The model under review builds one solid part; all positions refer to its coordinate system, in mm. A direction names the side the tool comes from. Coordinates: 2 decimals unless noted, no trailing zeros. Write each loop counter-clockwise with the first axis right and the second up, starting at its lowest first coordinate (ties: lowest second). Pieces come first, ordered by that corner, then holes.
1) Machinability: for faces 4 (the flat face through (70, 25, 8)), 5 (the flat face through (-8, 25, 70)), 6 (the flat face through (8, 25, -70)), 7 (the cylindrical face through (-57, 32, 0)), which of the approach directions +Z, -Z, +X, -X, +Y, -Y give a long, thin tool a straight path to every point of the face, cutting with its end or side? Answer none if there is none.
2) For P1, Ø10, axis at x = -51.5, y = 37.5, coming from the +Z side; P2, Ø3, axis at x = -57.5, y = 36.5, coming from the +Z side; P3, Ø4, axis at x = 14.5, y = 31, coming from the -Z side, all flat-tipped, find the tip position at first contact; note any pin that passes through.
3) Mouldability with a two-part tool opening along X and no side actions: class faces 1 (the cylindrical face through (79.845, 22.185, -41.53)), 2 (the flat face through (62, 42, -18.75)), 3 (the cylindrical face through (-19.524, 18.759, -4.336)) as released by +X, released by -X, zero draft, split by the parting line, or undercut.
4) Add section C-C, the plane z = 1. State the section outline as (x, y) points, then the cut area to 3 significant figures.
5) Add section A-A, the plane x = 0. State the section outline as (y, z) points, then the cut area to 3 significant figures.
6) Add section B-B, the plane y = 12. State the section outline as (x, z) points, then the cut area to 3 significant figures.
7) For line 1 (X direction, y = 9, z = 0); line 2 (X direction, y = 28, z = 0); line 3 (Z direction, x = 0, y = 40), list the stretches that pass through material, from the lowest coordinate up.
8) Add section D-D, the plane y = 32. State the section outline as (x, z) points, then the cut area to 3 significant figures.
from build123d import *

# Parameters (mm, degrees)
ESQUISSE1_R                  = 90
BOSS_EXTRU_1_DEPTH           = 45
ESQUISSE2_R                  = 9
ENL_V_MAT_EXTRU_1_DEPTH      = 45
ESQUISSE2_3_R                = 9
ENL_V_MAT_EXTRU_2_DEPTH      = 20
ENL_V_MAT_EXTRU_3_DEPTH      = 18.75
R_P_TITION_CIRCULAIRE2_COUNT = 4
ESQUISSE4_R                  = 30
ENL_V_MAT_EXTRU_4_DEPTH      = 8
ESQUISSE4_3_R                = 20
ENL_V_MAT_EXTRU_5_DEPTH      = 136


with BuildPart() as part:
    # Esquisse1 → Boss.-Extru.1 (new body)
    with BuildSketch(Plane(origin=(0, 0, 0), x_dir=(1, 0, 0), z_dir=(0, 1, 0))):
        with Locations(Location((0, 0, 0), (0, 0, 90))):
            Circle(ESQUISSE1_R)
    extrude(amount=BOSS_EXTRU_1_DEPTH)

    # Esquisse2 → Enl_v. mat.-Extru.1 (cut)
    with BuildSketch(Plane(origin=(0, 45, 0), x_dir=(1, 0, 0), z_dir=(0, 1, 0))):
        with Locations(Location((75, 0, 0), (0, 0, 270))):
            Circle(ESQUISSE2_R)
    enl_v_mat_extru_1 = extrude(amount=-ENL_V_MAT_EXTRU_1_DEPTH, mode=Mode.SUBTRACT)

    # Esquisse2_3 → Enl_v. mat.-Extru.2 (cut)
    with BuildSketch(Plane(origin=(0, 45, 0), x_dir=(1, 0, 0), z_dir=(0, 1, 0))):
        with BuildLine():
            Line((75, 18), (115, 18))
            ThreePointArc((115, 18), (133, 0), (115, -18))
            Line((115, -18), (75, -18))
            ThreePointArc((75, -18), (57, 0), (75, 18))
        make_face()
        with Locations(Location((75, 0, 0), (0, 0, 270))):
            Circle(ESQUISSE2_3_R, mode=Mode.SUBTRACT)
    enl_v_mat_extru_2 = extrude(amount=-ENL_V_MAT_EXTRU_2_DEPTH, mode=Mode.SUBTRACT)

    # Esquisse3 → Enl_v. mat.-Extru.3 (cut, symmetric)
    with BuildSketch(Plane.XY):
        Polygon((-0.90918463, 45), (101.87081537, 35.103411626), (101.87081537, 45), align=None)
    enl_v_mat_extru_3 = extrude(amount=ENL_V_MAT_EXTRU_3_DEPTH, both=True, mode=Mode.SUBTRACT)

    # Sym_trie1: Enl_v. mat.-Extru.3 across plane
    add(enl_v_mat_extru_3.mirror(Plane(origin=(0, 0, 0), x_dir=(0, 0, 1), z_dir=(1, 0, 0))), mode=Mode.SUBTRACT)

    # R_p_tition circulaire2: Enl_v. mat.-Extru.1, Enl_v. mat.-Extru.2 ×4 about axis
    r_p_tition_circulaire2_axis = Axis((0, 0, 0), (0, 1, 0))
    add([enl_v_mat_extru_1.rotate(r_p_tition_circulaire2_axis, i * 360 / R_P_TITION_CIRCULAIRE2_COUNT) for i in range(1, R_P_TITION_CIRCULAIRE2_COUNT)], mode=Mode.SUBTRACT)
    add([enl_v_mat_extru_2.rotate(r_p_tition_circulaire2_axis, i * 360 / R_P_TITION_CIRCULAIRE2_COUNT) for i in range(1, R_P_TITION_CIRCULAIRE2_COUNT)], mode=Mode.SUBTRACT)

    # Esquisse4 → Enl_v. mat.-Extru.4 (cut, symmetric)
    with BuildSketch(Plane(origin=(0, 45, 0), x_dir=(1, 0, 0), z_dir=(0, 1, 0))):
        with Locations(Location((0, 0, 0), (0, 0, 270))):
            Circle(ESQUISSE4_R)
    extrude(amount=ENL_V_MAT_EXTRU_4_DEPTH, both=True, mode=Mode.SUBTRACT)

    # Esquisse4_3 → Enl_v. mat.-Extru.5 (cut, through all)
    with BuildSketch(Plane(origin=(0, 45, 0), x_dir=(1, 0, 0), z_dir=(0, 1, 0))):
        with Locations(Location((0, 0, 0), (0, 0, 270))):
            Circle(ESQUISSE4_3_R)
    extrude(amount=-ENL_V_MAT_EXTRU_5_DEPTH, mode=Mode.SUBTRACT)


solid = part.part
Geometry results:
1. face 4: +X, +Y
1. face 5: +Z, +Y
1. face 6: -Z, +Y
1. face 7: -X, +Y
2. P1: stops at z = 77.06
2. P2: stops at z = 70.46
2. P3: stops at z = -67.81
3. face 1: split by the parting line
3. face 2: zero draft
3. face 3: undercut
4. outline: (-89.99, 0) - (-83.94, 0) - (-83.94, 25) - (-89.99, 25) - close; (-66.06, 0) - (-19.97, 0) - (-19.97, 37) - (-29.98, 37) - (-29.98, 42.03) - (-57.03, 39.42) - (-57.03, 25) - (-66.06, 25) - close; (19.97, 0) - (66.06, 0) - (66.06, 25) - (57.03, 25) - (57.03, 39.42) - (29.98, 42.03) - (29.98, 37) - (19.97, 37) - close; (83.94, 0) - (89.99, 0) - (89.99, 25) - (83.94, 25) - close
4. area: 3,700 mm2
5. outline: (0, -90) - (25, -90) - (25, -84) - (0, -84) - close; (0, -66) - (25, -66) - (25, -57) - (45, -57) - (45, -30) - (37, -30) - (37, -20) - (0, -20) - close; (0, 20) - (37, 20) - (37, 30) - (45, 30) - (45, 57) - (25, 57) - (25, 66) - (0, 66) - close; (0, 84) - (25, 84) - (25, 90) - (0, 90) - close
5. area: 3,920 mm2
6. outline: circle Ø180 at (0, 0); hole circle Ø18 at (-75, 0); hole circle Ø40 at (0, 0); hole circle Ø18 at (0, -75); hole circle Ø18 at (0, 75); hole circle Ø18 at (75, 0)
6. area: 23,200 mm2
7. line 1: x = -90 to -84, -66 to -20, 20 to 66, 84 to 90
7. line 2: x = -57 to -20, 20 to 57
7. line 3: z = -57 to -30, 30 to 57
8. outline: (-88.18, -18) arc R90 ccw to (-18, -88.18) - (-18, -75) arc R18 cw to (18, -75) - (18, -88.18) arc R90 ccw to (88.18, -18) - (75, -18) arc R18 cw to (75, 18) - (88.18, 18) arc R90 ccw to (18, 88.18) - (18, 75) arc R18 cw to (-18, 75) - (-18, 88.18) arc R90 ccw to (-88.18, 18) - (-75, 18) arc R18 cw to (-75, -18) - close; hole circle Ø40 at (0, 0)
8. area: 20,100 mm2
